Verification items for the finished model (mm, model axes). A direction names the side the tool comes from. Give positions to 0.01 mm unless a question says otherwise; leave off trailing zeros. Order: outer loops, then holes, each group sorted by start corner. A loop starts at its lowest first (then second) coordinate and runs counter-clockwise, first axis right, second up. Notation, with made-up numbers: (-4.75, 14.25) -> (8.25, 14.25) arc R19 ccw to (8.25, 47.25) -> close; hole circle Ø5 at (-9.75, 7.25). An arc over 180 degrees is marked (long way). Write each question's results on one line, items separated by ' | '. Start each with the question number.
1. Material ranges on L1, parallel to X at y = 12, z = 1.75; L2, parallel to Y at x = 22.5, z = 10.5; L3, parallel to Y at x = 22, z = 1.75, recorded low to high. Write a range as from..to.
2. Cross-section at D-D, the plane y = 20. Enter the section's corners in (x, z), then the cut area to 4 significant figures.
3. Cross-section at B-B, the plane x = 44. Enter the section's corners in (y, z), then the cut area to 3 significant figures.
4. Cross-section at A-A, the plane z = 17.25. Enter the section's corners in (x, y), then the cut area to 3 significant figures.
5. Set-up check for faces 1 (the face through (59.689, 9, 1)), 2 (the face through (38, 20, 2.5)), 3 (the face through (70.503, 18, 2)): record each of +Z, -Z, +X, -X, +Y, -Y from which the full face is reachable in a straight line by a thin tool's end or side.
6. Mould release check, pull along Y, two halves, no side actions. Record for faces 4 (the face through (7.103, 18, 2)), 5 (the face through (38, -4.36, 1)), 6 (the face through (16.51, 4.32, 1.23)): +Y half, -Y half, draft (parallel to the pull), parting line (faces both ways), or undercut.
7. Depth check by flat-ended pin: pin 1 Ø4 at (x, z) = (61.5, 15.5) entering from -Y; pin 2 Ø5 at (x, y) = (63, 13.72) entering from +Z. Enter the tip coordinate at first touch or a pass-through.
8. Cross-section at C-C, the plane y = 12.5. Enter the section's corners in (x, z).
from build123d import *

# Parameters (mm, degrees)
SKETCH_1_R          = 2
SKETCH_1_R_2        = 2.000000001
SKETCH_1_W          = 41.5
SKETCH_1_H          = 20.5
EXTRUDE_1_DEPTH     = 2.5
SKETCH_2_W          = 63.400042917
SKETCH_2_H          = 3
EXTRUDE_2_DEPTH     = 20
SKETCH_3_R          = 1.3
CUT_EXTRUDE_1_DEPTH = 3


with BuildPart() as part:
    # 草图1 → 凸台-拉伸1 (new body)
    with BuildSketch(Plane.XY):
        with BuildLine():
            Line((9.102779232, -4.360253516), (68.502822149, -4.360253516))
            ThreePointArc((68.502822149, -4.360253516), (69.917035712, -3.774467079), (70.502822149, -2.360253516))
            Line((70.502822149, -2.360253516), (70.502822149, 27.577468612))
            Line((70.502822149, 27.577468612), (7.102779232, 27.577468612))
            Line((7.102779232, 27.577468612), (7.102779232, -2.360253516))
            ThreePointArc((7.102779232, -2.360253516), (7.688565669, -3.774467079), (9.102779232, -4.360253516))
        make_face()
        with Locations((14.602780347, 13.71523364)):
            Circle(SKETCH_1_R, mode=Mode.SUBTRACT)
        with Locations((14.602779232, 3.71523364)):
            Circle(SKETCH_1_R, mode=Mode.SUBTRACT)
        with Locations((63.002822149, 3.71523364)):
            Circle(SKETCH_1_R_2, mode=Mode.SUBTRACT)
        with Locations((63.002821034, 13.71523364)):
            Circle(SKETCH_1_R, mode=Mode.SUBTRACT)
        with Locations((38.938588543, 8.81523364)):
            Rectangle(SKETCH_1_W, SKETCH_1_H, mode=Mode.SUBTRACT)
    extrude(amount=EXTRUDE_1_DEPTH)

    # 草图2 → 凸台-拉伸2 (add)
    with BuildSketch(Plane.XY.offset(2.5)):
        with Locations((38.802800691, 26.077468612)):
            Rectangle(SKETCH_2_W, SKETCH_2_H)
    extrude(amount=EXTRUDE_2_DEPTH)

    # 草图3 → 切除-拉伸1 (cut)
    with BuildSketch(Plane(origin=(0, 27.577468612, 0), x_dir=(1, 0, 0), z_dir=(0, 1, 0))):
        with Locations((13.80280069, -5.25)):
            Circle(SKETCH_3_R)
        with Locations((63.80280069, -5.25)):
            Circle(SKETCH_3_R)
        with Locations((63.80280069, -17.25)):
            Circle(SKETCH_3_R)
        with Locations((13.80280069, -17.25)):
            Circle(SKETCH_3_R)
    extrude(amount=-CUT_EXTRUDE_1_DEPTH, mode=Mode.SUBTRACT)


solid = part.part
Results below:
1) L1: x = 7.1..13.57, 15.63..18.19, 59.69..61.97, 64.03..70.5 | L2: y = 24.58..27.58 | L3: y = -4.36..-1.43, 19.07..27.58
2) outline: (7.1, 0) -> (70.5, 0) -> (70.5, 2.5) -> (7.1, 2.5) -> close | area: 158.5 mm²
3) outline: (-4.36, 0) -> (-1.43, 0) -> (-1.43, 2.5) -> (-4.36, 2.5) -> close; (19.07, 0) -> (27.58, 0) -> (27.58, 22.5) -> (24.58, 22.5) -> (24.58, 2.5) -> (19.07, 2.5) -> close | area: 88.6 mm²
4) outline: (7.1, 24.58) -> (12.5, 24.58) -> (12.5, 27.58) -> (7.1, 27.58) -> close; (15.1, 24.58) -> (62.5, 24.58) -> (62.5, 27.58) -> (15.1, 27.58) -> close; (65.1, 24.58) -> (70.5, 24.58) -> (70.5, 27.58) -> (65.1, 27.58) -> close | area: 175 mm²
5) face 1: +Z, -Z | face 2: +Z, +X, -X, -Y | face 3: +Z, -Z, +X, +Y, -Y
6) face 4: draft | face 5: -Y half | face 6: undercut
7) pin 1: stops at y = 24.58 | pin 2: stops at z = 2.5
8) outline: (7.1, 0) -> (13.01, 0) -> (13.01, 2.5) -> (7.1, 2.5) -> close; (16.19, 0) -> (18.19, 0) -> (18.19, 2.5) -> (16.19, 2.5) -> close; (59.69, 0) -> (61.41, 0) -> (61.41, 2.5) -> (59.69, 2.5) -> close; (64.59, 0) -> (70.5, 0) -> (70.5, 2.5) -> (64.59, 2.5) -> close
